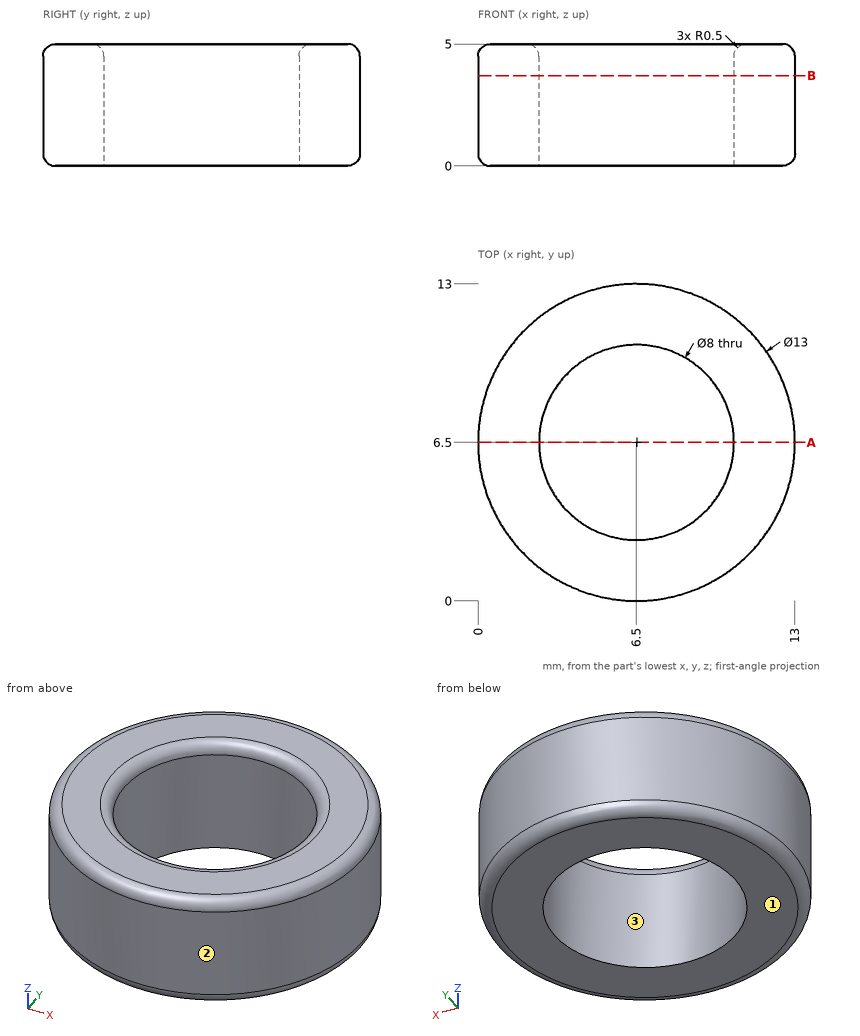
Job drawing, mm, ordinate dimensions from the low corner. One solid piece. Coordinates: 2 decimals unless noted, no trailing zeros. Order: outer loops, then holes, each group sorted by start corner. A loop starts at its lowest first (then second) coordinate and runs counter-clockwise, first axis right, second up. Notation, with made-up numbers: (-12, 57.25) - (44, 57.25) arc R19 cw to (44, 93.25) - close; hole circle Ø2 at (-6, 5.25). An arc over 180 degrees is marked (long way). Return JSON: item names as keys, results as strings. Group by question number.
1) Mould opens along X. For the marked faces 1, 2 and 3 say: released by +X, released by -X, zero draft, split by the parting line, or undercut.
2) Flat gauge pin, fed straight in: P1, Ø1, axis at y = 2.5, z = 3, coming from the -X side. Where does the tip first touch, or does it go through?
3) Probe line 1 (Y direction, x = 6.5, z = 3.3); line 2 (Y direction, x = 4.25, z = 2.1); line 3 (X direction, y = 9, z = 3.9). List the from-to ranges inside material, lowest first. Write a range as from..to.
4) Saw through at A-A, the plane y = 6.5. Write the cut outline in (x, z).
5) Saw through at B-B, the plane z = 3.7. Write the cut outline in (x, y).
Values found:
{
 "1": {"face 1": "zero draft", "face 2": "split by the parting line", "face 3": "undercut"},
 "2": {"P1": "stops at x = 1.02"},
 "3": {"line 1": "y = 0..2.5, 10.5..13", "line 2": "y = 0.4..3.19, 9.81..12.6", "line 3": "x = 0.5..3.38, 9.62..12.5"},
 "4": {"outline": "(0, 0.5) arc R0.5 ccw to (0.5, 0) - (2.5, 0) - (2.5, 4.5) arc R0.5 ccw to (2, 5) - (0.5, 5) arc R0.5 ccw to (0, 4.5) - close; (10.5, 0) - (12.5, 0) arc R0.5 ccw to (13, 0.5) - (13, 4.5) arc R0.5 ccw to (12.5, 5) - (11, 5) arc R0.5 ccw to (10.5, 4.5) - close"},
 "5": {"outline": "circle Ø13 at (6.5, 6.5); hole circle Ø8 at (6.5, 6.5)"}
}
